```python
from build123d import *

# Parameters (mm, degrees)
SKETCH_1_W          = 120
SKETCH_1_H          = 36
SKETCH_1_R          = 0.85
SKETCH_1_R_2        = 1.6
EXTRUDE_1_DEPTH     = 3
CUT_EXTRUDE_1_DEPTH = 1.5
FILLET_1_R          = 5


with BuildPart() as part:
    # 草图1 → 凸台-拉伸1 (new body)
    with BuildSketch(Plane.XY):
        with Locations((60, 18)):
            Rectangle(SKETCH_1_W, SKETCH_1_H)
        with Locations((48.686291501, 29.313708499)):
            Circle(SKETCH_1_R, mode=Mode.SUBTRACT)
        with Locations((48.686291501, 6.686291501)):
            Circle(SKETCH_1_R, mode=Mode.SUBTRACT)
        with Locations(Location((71.313708499, 6.686291501, 0), (0, 0, 180))):
            Circle(SKETCH_1_R, mode=Mode.SUBTRACT)
        with Locations(Location((71.313708499, 29.313708499, 0), (0, 0, 180))):
            Circle(SKETCH_1_R, mode=Mode.SUBTRACT)
        with Locations((60, 29.313708499)):
            Circle(SKETCH_1_R_2, mode=Mode.SUBTRACT)
        with Locations(Location((48.686291501, 18, 0), (0, 0, 180))):
            Circle(SKETCH_1_R_2, mode=Mode.SUBTRACT)
        with Locations((60, 6.686291501)):
            Circle(SKETCH_1_R_2, mode=Mode.SUBTRACT)
        with Locations(Location((71.313708499, 18, 0), (0, 0, 180))):
            Circle(SKETCH_1_R_2, mode=Mode.SUBTRACT)
        with BuildLine():
            Line((56.604710662, 30.671392317), (56.28868628, 31.850811367))
            ThreePointArc((56.28868628, 31.850811367), (49.860502354, 28.139497646), (46.149188633, 21.71131372))
            Line((46.149188633, 21.71131372), (47.328607683, 21.395289338))
            Line((47.328607683, 21.395289338), (56.604710662, 30.671392317))
        make_face(mode=Mode.SUBTRACT)
        with BuildLine():
            Line((63.395289338, 30.671392317), (63.71131372, 31.850811367))
            ThreePointArc((63.71131372, 31.850811367), (70.139497646, 28.139497646), (73.850811367, 21.71131372))
            Line((73.850811367, 21.71131372), (72.671392317, 21.395289338))
            Line((72.671392317, 21.395289338), (63.395289338, 30.671392317))
        make_face(mode=Mode.SUBTRACT)
        with BuildLine():
            Line((63.395289338, 5.328607683), (63.71131372, 4.149188633))
            ThreePointArc((63.71131372, 4.149188633), (70.139497646, 7.860502354), (73.850811367, 14.28868628))
            Line((73.850811367, 14.28868628), (72.671392317, 14.604710662))
            Line((72.671392317, 14.604710662), (63.395289338, 5.328607683))
        make_face(mode=Mode.SUBTRACT)
        with BuildLine():
            Line((47.328607683, 14.604710662), (46.149188633, 14.28868628))
            ThreePointArc((46.149188633, 14.28868628), (49.860502354, 7.860502354), (56.28868628, 4.149188633))
            Line((56.28868628, 4.149188633), (56.604710662, 5.328607683))
            Line((56.604710662, 5.328607683), (47.328607683, 14.604710662))
        make_face(mode=Mode.SUBTRACT)
    extrude(amount=EXTRUDE_1_DEPTH)

    # 草图2 → 切除-拉伸1 (cut)
    with BuildSketch(Plane.XY.offset(3)):
        Polygon((2.3, 30.05), (18, 30.05), (18, 35), (20.9, 35), (20.9, 30.05), (29.8, 30.05), (29.8, 14.97), (25.2, 14.97), (25.2, 7.55), (20.9, 7.55), (20.9, 2.6), (18, 2.6), (18, 7.45), (2.3, 7.45), align=None)
        Polygon((117.7, 30.05), (102, 30.05), (102, 35), (99.1, 35), (99.1, 30.05), (90.2, 30.05), (90.2, 14.97), (94.8, 14.97), (94.8, 7.55), (99.1, 7.55), (99.1, 2.6), (102, 2.6), (102, 7.45), (117.7, 7.45), align=None)
    extrude(amount=-CUT_EXTRUDE_1_DEPTH, mode=Mode.SUBTRACT)

    # 圆角1
    fillet_1_edges = [part.edges().sort_by_distance(p)[0] for p in [
        (0, 36, 1.5),
        (120, 36, 1.5),
        (120, 0, 1.5),
        (0, 0, 1.5),
    ]]
    fillet(fillet_1_edges, radius=FILLET_1_R)


solid = part.part
```
Check sheet for the modelled part. Datum: model origin and axes. Units: mm. A direction names the side the tool comes from. Give positions to 0.01 mm unless a question says otherwise; leave off trailing zeros. Write each loop counter-clockwise with the first axis right and the second up, starting at its lowest first coordinate (ties: lowest second). Pieces come first, ordered by that corner, then holes.
Item 1: Draft check along Y on faces 3 (the face through (0, 18, 1)), 4 (the face through (49.786, 7.935, 1.479)), 5 (the face through (72.912, 17.93, 1.479)), 6 (the face through (118, 1, 2)). Enter one of: released by +Y, released by -Y, zero draft, split by the parting line, or undercut.
Item 2: Cross-section at C-C (z = 1.05). Count the separate pieces of the cut face and the enclosed holes in it, and give its area (3 significant figures).
Item 3: Cross-section at A-A (x = 60). Enter the section's corners in (y, z).
Item 4: Cross-section at B-B (y = 18). Enter the section's corners in (x, z), and give its area (3 significant figures).
Item 5: Access from +Z, -Z, +X, -X, +Y, -Y to the whole of each face (thin tool, end or side, straight path). Record for faces 1 (the face through (59, 18, 3)), 2 (the face through (68.098, 25.968, 1.479)).
Item 6: Gauge pin test, flat end, axial feed: pin 1 (8 mm diameter, centred on x = 16.5, y = 20, fed in from +Z). Record the tip position at first contact, or that the pin passes through.
Item 7: Cross-section at D-D (y = 10). Enter the section's corners in (x, z), and give its area (3 significant figures).
Item 8: Scan lines: L1, parallel to X at y = 18, z = 1.35; L2, parallel to X at y = 15.5, z = 2.35; L3, parallel to Y at x = 53, z = 2.55. Record each from-to range of solid material in increasing order.
Report:
1. face 3: zero draft
1. face 4: undercut
1. face 5: undercut
1. face 6: released by -Y
2. separate pieces: 1
2. enclosed holes: 12
2. area: 4,120 mm2
3. outline: (0, 0) - (5.09, 0) - (5.09, 3) - (0, 3) - close; (8.29, 0) - (27.71, 0) - (27.71, 3) - (8.29, 3) - close; (30.91, 0) - (36, 0) - (36, 3) - (30.91, 3) - close
4. outline: (0, 0) - (47.09, 0) - (47.09, 3) - (29.8, 3) - (29.8, 1.5) - (2.3, 1.5) - (2.3, 3) - (0, 3) - close; (50.29, 0) - (69.71, 0) - (69.71, 3) - (50.29, 3) - close; (72.91, 0) - (120, 0) - (120, 3) - (117.7, 3) - (117.7, 1.5) - (90.2, 1.5) - (90.2, 3) - (72.91, 3) - close
4. area: 258 mm2
5. face 1: +Z, +X, -X, +Y, -Y
5. face 2: +Z, -Z
6. pin 1: stops at z = 1.5
7. outline: (0, 0) - (48.1, 0) - (48.1, 3) - (25.2, 3) - (25.2, 1.5) - (2.3, 1.5) - (2.3, 3) - (0, 3) - close; (51.93, 0) - (68.07, 0) - (68.07, 3) - (51.93, 3) - close; (71.9, 0) - (120, 0) - (120, 3) - (117.7, 3) - (117.7, 1.5) - (94.8, 1.5) - (94.8, 3) - (71.9, 3) - close
7. area: 268 mm2
8. L1: x = 0 to 47.09, 50.29 to 69.71, 72.91 to 120
8. L2: x = 0 to 2.3, 29.8 to 90.2, 117.7 to 120
8. L3: y = 0 to 5.49, 8.93 to 27.07, 30.51 to 36
